Part model, mm, in its own coordinate system. Face numbers are marked on the shaded views. Round coordinates to 2 decimals unless told otherwise and drop trailing zeros. Loops run counter-clockwise (first coordinate to the right, second up) from the corner with the lowest first, then second, coordinate; pieces in that order, holes last.
(1) Cut at A-A on z = -6. List the corners of the cut face in (x, y).
(2) Cut at B-B on y = 1.75. List the corners of the cut face in (x, z), then the cut area to 3 significant figures.
(3) Mould opens along Z. For the marked faces 1, 2 and 3 say: +Z half, -Z half, draft (parallel to the pull), parting line (faces both ways), or undercut.
(4) Flat gauge pins, fed straight in: pin 1 (1.6 mm diameter, centred on x = -11.5, y = 4.5, fed in from +Z); pin 2 (2.5 mm diameter, centred on x = -20.41, z = -31, fed in from +Y); pin 3 (1.6 mm diameter, centred on x = -42, y = 3.5, fed in from -Z); pin 4 (1 mm diameter, centred on y = 4.5, z = -22, fed in from -X). Where does each tip first touch, or does it go through?
(5) Cut at C-C on x = -36. List the corners of the cut face in (y, z).
(6) Cut at D-D on x = -4. List the corners of the cut face in (y, z), then the cut area to 3 significant figures.
(7) Probe probe 1 along X at (y, z) = (4, -42); probe 2 along Z at (x, y) = (-4, 4); probe 3 along Y at (x, z) = (-12, -41.5). List the from-to ranges inside material, lowest first.
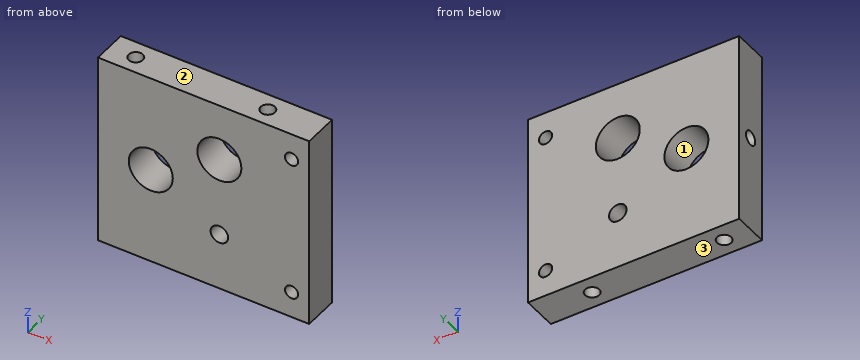
Autodesk Inventor part; units mm, degrees
ref_plane "Arbeitsebene1" through (0, 0, -22) normal (0, 0, 1) x (1, 0, 0)
ref_plane "YZ Plane" through (0, 0, 0) normal (1, 0, 0) x (0, 1, 0)
ref_plane "XZ Plane" through (0, 0, 0) normal (0, 1, 0) x (-1, 0, 0)
sketch "Skizze1" plane through (0, 0, 0) normal (0, 1, 0) x (-1, 0, 0)
  line L0 (0, 0) -> (48, 0)
  line L1 (48, 0) -> (48, -44)
  line L2 (48, -44) -> (0, -44)
  line L3 (0, -44) -> (0, 0)
  dimension "d0" = 44
  dimension "d1" = 48
extrude "Extrusion1" add sketch "Skizze1" along normal blind 8
sketch "Skizze2" plane through (0, 8, 0) normal (0, 1, 0) x (1, 0, 0)
  circle A0 centre (-36, 22) radius 5
  circle A1 centre (-20.4115, 13) radius 5
  circle A2 centre (-20.4115, 31) radius 2
  line L0 (0, 0) -> (0, 44)
  line L1 (0, 22) -> (-47.9314, 22) construction
  line L2 (-48, 44) -> (-48, 0)
  dimension "d4" = 9
  dimension "d5" = 12
  dimension "d6" = 10
  dimension "d7" = 18
  dimension "d8" = 10
  dimension "d9" = 4
extrude "Extrusion2" cut sketch "Skizze2" against normal up to surface (8 mm away)
sketch "Skizze3" plane through (-48, 0, -44) normal (-1, 0, 0) x (0, 0, 1)
  line L0 (44, 0) -> (44, 8)
  line L1 (0, 0) -> (44, 0)
  point P0 (22, 4)
  point P1 (44, 4)
  point P2 (22, 0)
hole "Bohrung1" at (-48, 4, -22) direction (1, 0, 0) diameter 3.242 depth 4
sketch "Skizze4" plane through (0, 8, 0) normal (0, 1, 0) x (1, 0, 0)
  line L0 (0, 0) -> (0, 44)
  line L1 (-48, 0) -> (0, 0)
  point P0 (-4, 6)
  point P1 (-4, 38)
  dimension "d26" = 4
  dimension "d27" = 6
  dimension "d28" = 32
hole "Bohrung2" at (-4, 8, -6) at (-4, 8, -38) direction (0, -1, 0) diameter 3 depth 8
sketch "Skizze5" plane through (0, 0, -44) normal (0, 0, -1) x (-1, 0, 0)
  line L0 (48, 0) -> (48, 8)
  line L1 (0, 0) -> (0, 8)
  point P0 (12, 4)
  point P1 (42, 4)
  point P2 (48, 4)
  dimension "d36" = 30
  dimension "d37" = 12
hole "Bohrung3" at (-12, 4, -44) at (-42, 4, -44) direction (0, 0, 1) diameter 3.242 depth 10
ref_plane "Arbeitsebene1" through (0, 0, -22) normal (0, 0, 1) x (1, 0, 0)
mirror "Spiegeln1" about plane through (0, 0, -22) normal (0, 0, 1) of "Bohrung3"
properties part number "1015"
Final values:
1. outline: (-48, 0) - (-5.5, 0) - (-5.5, 8) - (-48, 8) - close; (-2.5, 0) - (0, 0) - (0, 8) - (-2.5, 8) - close; hole circle Ø3.24 at (-42, 4); hole circle Ø3.24 at (-12, 4)
2. outline: (-48, -44) - (0, -44) - (0, 0) - (-48, 0) - close; hole circle Ø10 at (-36, -22); hole circle Ø10 at (-20.41, -13); hole circle Ø4 at (-20.41, -31); hole circle Ø3 at (-4, -38); hole circle Ø3 at (-4, -6)
2. area: 1,930 mm2
3. face 1: undercut
3. face 2: +Z half
3. face 3: -Z half
4. pin 1: stops at z = -10
4. pin 2: passes through
4. pin 3: stops at z = -34
4. pin 4: stops at x = -44
5. outline: (0, -44) - (8, -44) - (8, -27) - (0, -27) - close; (0, -17) - (8, -17) - (8, 0) - (0, 0) - close
6. outline: (0, -44) - (8, -44) - (8, -39.5) - (0, -39.5) - close; (0, -36.5) - (8, -36.5) - (8, -7.5) - (0, -7.5) - close; (0, -4.5) - (8, -4.5) - (8, 0) - (0, 0) - close
6. area: 304 mm2
7. probe 1: x = -48 to -43.62, -40.38 to -13.62, -10.38 to 0
7. probe 2: z = -44 to -39.5, -36.5 to -7.5, -4.5 to 0
7. probe 3: y = 0 to 2.38, 5.62 to 8
